from build123d import *

# Parameters (mm, degrees)
F4_W         = 12
F4_H         = 14
F4_R         = 2.75
F0_DEPTH     = 6
F5_DEPTH     = 3.5
F2_R         = 0.2
F3_T1_DEPTH  = 13.6
F3_S5_W      = 0.2
F3_S5_H      = 0.2
F3_T6_DEPTH  = 0.2
F3_S11_W     = 0.2
F3_S11_H     = 0.2
F3_T12_DEPTH = 0.2


# Not quite as in the source:
# - a fillet or chamfer that OpenCascade refuses, or shapes differently, is made with other operations: its cross-section is extruded or revolved along the edge and cut away or added


with BuildPart() as f0:
    # F4 (on Top) → F0 (new body)
    with BuildSketch(Plane.XY):
        with Locations((6, 2.0147956188)):
            Rectangle(F4_W, F4_H)
        with Locations((6, 2.0147956188)):
            Circle(F4_R, mode=Mode.SUBTRACT)
    extrude(amount=F0_DEPTH)

    # F1 (on face) → F5 (cut)
    with BuildSketch(Plane.XY.offset(6)):
        Polygon((4.015, -1.4233252342), (7.985, -1.4233252342), (9.97, 2.0147956188), (7.985, 5.4529164718), (4.015, 5.4529164718), (2.03, 2.0147956188), align=None)
    extrude(amount=-F5_DEPTH, mode=Mode.SUBTRACT)

    # F2
    f2_edges = [f0.edges().sort_by_distance(p)[0] for p in [
        (6, -4.985204, 6),
        (0, 2.014796, 6),
        (6, 9.014796, 6),
        (12, 2.014796, 6),
        (6, 5.452916, 6),
        (8.9775, 3.733856, 6),
        (8.9775, 0.295735, 6),
        (6, -1.423325, 6),
        (3.0225, 0.295735, 6),
        (3.0225, 3.733856, 6),
        (3.25, 2.014796, 2.5),
        (12, -4.985204, 3),
        (12, 9.014796, 3),
        (12, 2.014796, 0),
        (6, -4.985204, 0),
        (0, -4.985204, 3),
        (3.25, 2.014796, 0),
        (6, 9.014796, 0),
        (0, 9.014796, 3),
    ]]
    fillet(f2_edges, radius=F2_R)

    # F3: fillet of radius 0.2 on 1 edges, made by hand

    # F3_s2 → F3_t1 (cut)
    with BuildSketch(Plane.XZ.offset(-8.8147956188)):
        with BuildLine():
            ThreePointArc((0, 0.2), (0.0585786438, 0.0585786438), (0.2, 0))
            Line((0.2, 0), (0, 0))
            Line((0, 0), (0, 0.2))
        make_face()
    extrude(amount=F3_T1_DEPTH, mode=Mode.SUBTRACT)


with BuildPart() as f3_tool4:
    # F3_s5 → F3_t6 (new body)
    with BuildSketch(Plane.YZ.offset(0.2)):
        with Locations((8.9147956188, 0.1)):
            Rectangle(F3_S5_W, F3_S5_H)
    extrude(amount=-F3_T6_DEPTH)

    # F3_s7 → F3_t8 (revolve, cut)
    with BuildSketch(Plane(origin=(0.2, 8.8147956188, 0.2), x_dir=(0, -0.7071067812, 0.7071067812), z_dir=(0, -0.7071067812, -0.7071067812))):
        with BuildLine():
            ThreePointArc((0, -0.2), (0.2, 0), (0, 0.2))
            Line((0, 0.2), (0, -0.2))
        make_face()
    revolve(axis=Axis((0.2, 8.8147956188, 0.2), (-1, 0, 0)), mode=Mode.SUBTRACT)


with BuildPart() as f0_1:
    add(f0.part)

    # F3_t3: cut F3_tool4
    add(f3_tool4.part, mode=Mode.SUBTRACT)


with BuildPart() as f3_tool10:
    # F3_s11 → F3_t12 (new body)
    with BuildSketch(Plane.YZ.offset(0.2)):
        with Locations((-4.8852043812, 0.1)):
            Rectangle(F3_S11_W, F3_S11_H)
    extrude(amount=-F3_T12_DEPTH)

    # F3_s13 → F3_t14 (revolve, cut)
    with BuildSketch(Plane(origin=(0.2, -4.7852043812, 0.2), x_dir=(0, 0.7071067812, 0.7071067812), z_dir=(0, -0.7071067812, 0.7071067812))):
        with BuildLine():
            ThreePointArc((0, -0.2), (0.2, 0), (0, 0.2))
            Line((0, 0.2), (0, -0.2))
        make_face()
    revolve(axis=Axis((0.2, -4.7852043812, 0.2), (-1, 0, 0)), mode=Mode.SUBTRACT)


with BuildPart() as f0_2:
    add(f0_1.part)

    # F3_t9: cut F3_tool10
    add(f3_tool10.part, mode=Mode.SUBTRACT)


solid = f0_2.part
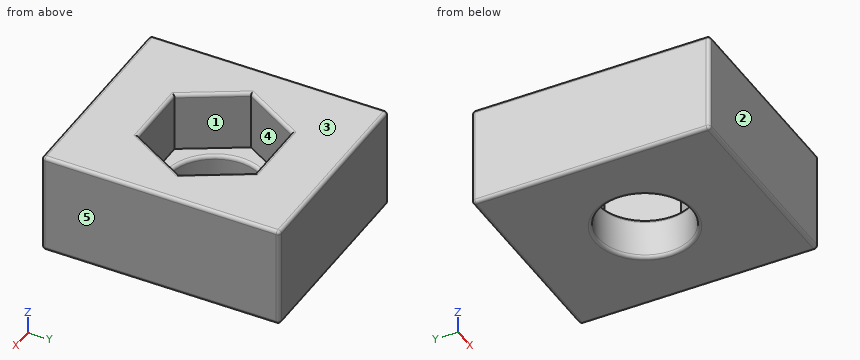
Input: part model. Units: mm. Frame: model coordinates. Face numbers are marked on the shaded views. A direction names the side the tool comes from. Give positions to 0.01 mm unless a question says otherwise; leave off trailing zeros. Loops run counter-clockwise (first coordinate to the right, second up) from the corner with the lowest first, then second, coordinate; pieces in that order, holes last. Notation, with made-up numbers: (69.25, 80) -> (127.25, 80) arc R17 ccw to (127.25, 106) -> close; hole circle Ø2 at (-18.5, -37). An arc over 180 degrees is marked (long way). Answer as a JSON object with one key per item and string values. Group by question number.
Item 1: Cut plane A-A, the plane z = 1.1. Return the cut outline in (x, y), and give its area (3 significant figures).
Item 2: Line query: probe 1 along Y at (x, z) = (6, 1.65); probe 2 along X at (y, z) = (0.25, 4.5); probe 3 along Y at (x, z) = (5, 4.3). Output: solid intervals per line, ascending.
Item 3: Cut plane C-C, the plane z = 3.85. Return the cut outline in (x, y) (3 decimals), and give its area (3 significant figures).
Item 4: Reachability of the marked faces 1 and 2 from +Z, -Z, +X, -X, +Y, -Y: full face, straight path, thin tool, end or side. Return the list, or none.
Item 5: Pull-direction query (X, two-part tool) for the marked faces 3, 4 and 5; classes: released by +X, released by -X, zero draft, split by the parting line, or undercut.
Item 6: Pin query (flat end, axial travel): P1, Ø2, axis at x = 6.5, y = 2.5, coming from the +Z side; P2, Ø6.5, axis at x = 6, y = 2.01, coming from the +Z side. Return the tip coordinate at first contact, or that it passes through.
Item 7: Cut plane B-B, the plane x = 6. Return the cut outline in (y, z), and give its area (3 significant figures).
Checks:
{
 "1": {"outline": "(0, -4.79) arc R0.2 ccw to (0.2, -4.99) -> (11.8, -4.99) arc R0.2 ccw to (12, -4.79) -> (12, 8.81) arc R0.2 ccw to (11.8, 9.01) -> (0.2, 9.01) arc R0.2 ccw to (0, 8.81) -> close; hole circle Ø5.5 at (6, 2.01)", "area": "144 mm²"},
 "2": {"probe 1": "y = -4.99 to -0.74, 4.76 to 9.01", "probe 2": "x = 0 to 3.05, 8.95 to 12", "probe 3": "y = -4.99 to -1.42, 5.45 to 9.01"},
 "3": {"outline": "(0, -4.785) arc R0.2 ccw to (0.2, -4.985) -> (11.8, -4.985) arc R0.2 ccw to (12, -4.785) -> (12, 8.815) arc R0.2 ccw to (11.8, 9.015) -> (0.2, 9.015) arc R0.2 ccw to (0, 8.815) -> close; hole (2.03, 2.015) -> (4.015, -1.423) -> (7.985, -1.423) -> (9.97, 2.015) -> (7.985, 5.453) -> (4.015, 5.453) -> close", "area": "127 mm²"},
 "4": {"face 1": "+Z", "face 2": "+Z, -Z, +X, -X, -Y"},
 "5": {"face 3": "zero draft", "face 4": "undercut", "face 5": "released by +X"},
 "6": {"P1": "passes through", "P2": "stops at z = 2.5"},
 "7": {"outline": "(-4.99, 0.2) arc R0.2 ccw to (-4.79, 0) -> (-0.94, 0) arc R0.2 ccw to (-0.74, 0.2) -> (-0.74, 2.3) arc R0.2 ccw to (-0.94, 2.5) -> (-1.42, 2.5) -> (-1.42, 5.8) arc R0.2 ccw to (-1.62, 6) -> (-4.79, 6) arc R0.2 ccw to (-4.99, 5.8) -> close; (4.76, 0.2) arc R0.2 ccw to (4.96, 0) -> (8.81, 0) arc R0.2 ccw to (9.01, 0.2) -> (9.01, 5.8) arc R0.2 ccw to (8.81, 6) -> (5.65, 6) arc R0.2 ccw to (5.45, 5.8) -> (5.45, 2.5) -> (4.96, 2.5) arc R0.2 ccw to (4.76, 2.3) -> close", "area": "46.1 mm²"}
}
